Answer from the drawing. Dimensions are ordinates in mm from the lowest x, y and z of the part. Coordinates: 2 decimals unless noted, no trailing zeros. Write each loop counter-clockwise with the first axis right and the second up, starting at its lowest first coordinate (ties: lowest second). Pieces come first, ordered by that corner, then holes. Notation, with made-up numbers: (60.25, -23.5) -> (99.25, -23.5) arc R9 ccw to (99.25, -8.5) -> close; hole circle Ø6 at (-23.75, 54). An arc over 180 degrees is marked (long way). Answer as a JSON object with one key per item and string values. Group by question number.
(1) Straight lines are drawn through the part: L1, parallel to X at y = 101.5, z = 0.6; L2, parallel to Y at x = 15, z = 0.7; L3, parallel to Y at x = 9.75, z = 0.8. For each, find the intervals that lie inside material, in ascending order.
(2) Find section B-B (x = 22.5). Give the vertices of the cut face in (y, z), then the cut area to 3 significant figures.
(3) A flat-ended cylindrical pin translates along its axis: P1, Ø8, axis at x = 18, y = 66.5, coming from the -Z side. Find the tip coordinate at first contact, or state that the pin passes through.
(4) Find section C-C (z = 0.8). Give the vertices of the cut face in (x, y), then the cut area to 3 significant figures.
(5) Find section A-A (y = 134). Give the vertices of the cut face in (x, z).
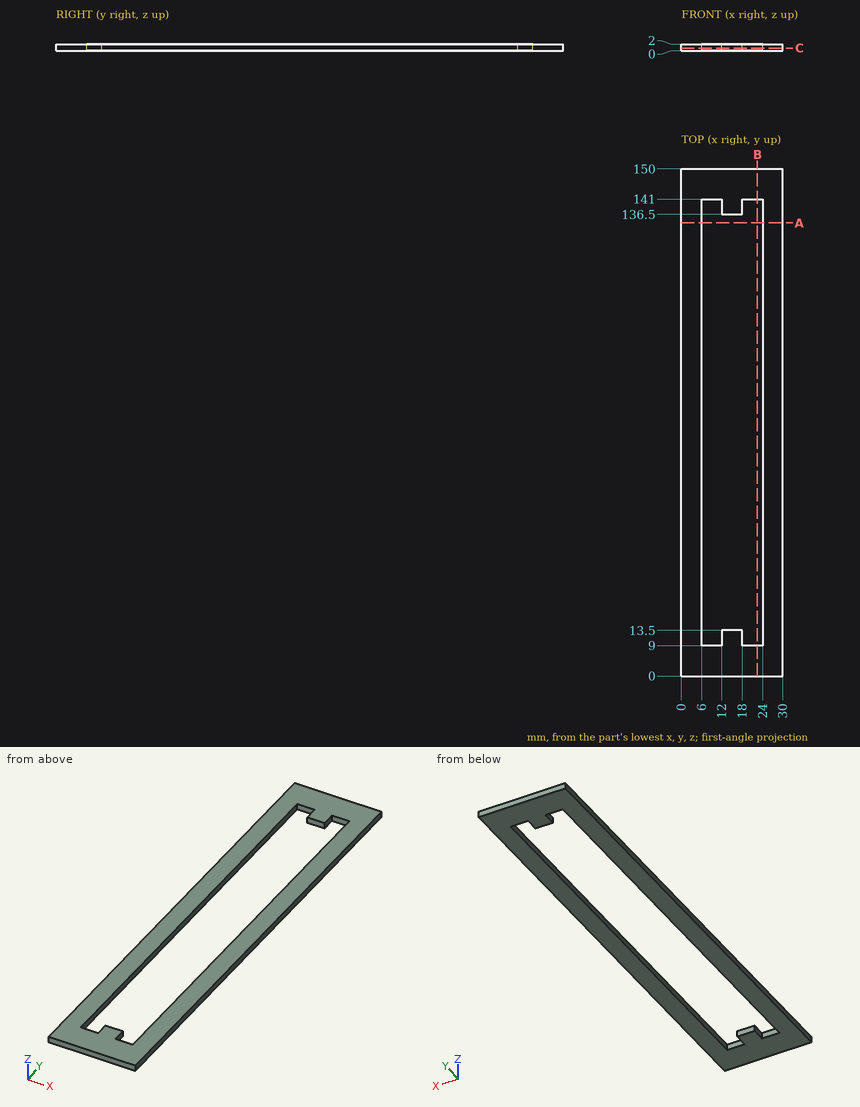
Results below:
{
 "1": {"L1": "x = 0 to 6, 24 to 30", "L2": "y = 0 to 13.5, 136.5 to 150", "L3": "y = 0 to 9, 141 to 150"},
 "2": {"outline": "(0, 0) -> (9, 0) -> (9, 2) -> (0, 2) -> close; (141, 0) -> (150, 0) -> (150, 2) -> (141, 2) -> close", "area": "36.0 mm2"},
 "3": {"P1": "passes through"},
 "4": {"outline": "(0, 0) -> (30, 0) -> (30, 150) -> (0, 150) -> close; hole (6, 9) -> (12, 9) -> (12, 13.5) -> (18, 13.5) -> (18, 9) -> (24, 9) -> (24, 141) -> (18, 141) -> (18, 136.5) -> (12, 136.5) -> (12, 141) -> (6, 141) -> close", "area": "2,180 mm2"},
 "5": {"outline": "(0, 0) -> (6, 0) -> (6, 2) -> (0, 2) -> close; (24, 0) -> (30, 0) -> (30, 2) -> (24, 2) -> close"}
}
